The listing builds one solid part. Answer for the finished solid, in the listing's coordinates (mm). Give positions to 0.01 mm unless a question says otherwise; leave off trailing zeros. Loops run counter-clockwise (first coordinate to the right, second up) from the corner with the lowest first, then second, coordinate; pieces in that order, holes last. Notation, with made-up numbers: (6.25, 6) - (61.25, 6) arc R19 cw to (61.25, 14) - close; hole circle Ø10 at (-16.5, 17). An arc over 180 degrees is marked (long way). Write item = value, one per line. Start each with the question number.
1) The part is cut by section A-A on y = 0. Write down the section's boundary in (x, z), plus the area to 3 significant figures.
2) The part is cut by section B-B on x = 0. Write down the section's boundary in (y, z).
3) Consider probe 1 along X at (y, z) = (-0.5, 10.5); probe 2 along Y at (x, z) = (0, -0.8); probe 3 along Z at (x, y) = (69, 3). Determine where each line is inside the solid, lowest interval first.
4) The part is cut by section D-D on x = -21. Write down the section's boundary in (y, z).
5) The part is cut by section C-C on z = 3.5. Write down the section's boundary in (x, y), plus the area to 3 significant figures.
6) Flat-ended cylindrical pins translate along their axes: P1, Ø3, axis at x = 51.5, y = -1, coming from the +Z side; P2, Ø6, axis at x = 32.5, z = 3.5, coming from the -Y side. Find the tip coordinate at first contact, or state that the pin passes through.
from build123d import *

# Parameters (mm, degrees)
BOSS_EXTRUDE1_DEPTH     = 3.5
SKETCH3_R               = 2
CUT_EXTRUDE1_DEPTH      = 7
SKETCH4_R               = 1.5
CUT_EXTRUDE2_DEPTH      = 1
CUT_EXTRUDE2_DEPTH_BACK = 190


with BuildPart() as part:
    # Sketch1 → Boss-Extrude1 (new body, symmetric)
    with BuildSketch(Plane(origin=(0, 0, 0), x_dir=(1, 0, 0), z_dir=(0, 1, 0))):
        Polygon((94.5, 1.75), (94.5, -20), (91, -20), (91, -1.75), (-91, -1.75), (-91, -20), (-94.5, -20), (-94.5, 1.75), align=None)
    extrude(amount=BOSS_EXTRUDE1_DEPTH, both=True)

    # Sketch3 → Cut-Extrude1 (cut)
    with BuildSketch(Plane(origin=(0, 0, -1.75), x_dir=(-1, 0, 0), z_dir=(0, 0, -1))):
        Circle(SKETCH3_R)
    extrude(amount=-CUT_EXTRUDE1_DEPTH, mode=Mode.SUBTRACT)

    # Sketch4 → Cut-Extrude2 (cut, two sides)
    with BuildSketch(Plane.ZY.offset(94.5)) as cut_extrude2_sk:
        with Locations((16.25, 0)):
            Circle(SKETCH4_R)
    extrude(amount=CUT_EXTRUDE2_DEPTH, mode=Mode.SUBTRACT)
    extrude(cut_extrude2_sk.sketch, amount=-CUT_EXTRUDE2_DEPTH_BACK, mode=Mode.SUBTRACT)


solid = part.part
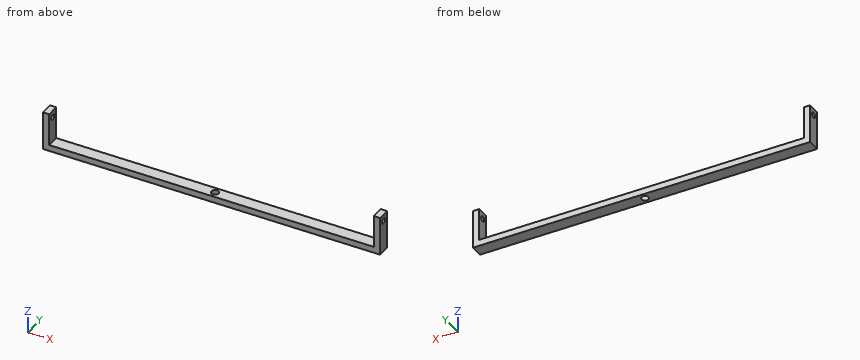
Answer below:
q1.outline = (-94.5, -1.75) - (-2, -1.75) - (-2, 1.75) - (-91, 1.75) - (-91, 14.75) - (-94.5, 14.75) - close; (-94.5, 17.75) - (-91, 17.75) - (-91, 20) - (-94.5, 20) - close; (2, -1.75) - (94.5, -1.75) - (94.5, 14.75) - (91, 14.75) - (91, 1.75) - (2, 1.75) - close; (91, 17.75) - (94.5, 17.75) - (94.5, 20) - (91, 20) - close
q1.area = 754 mm2
q2.outline = (-3.5, -1.75) - (-2, -1.75) - (-2, 1.75) - (-3.5, 1.75) - close; (2, -1.75) - (3.5, -1.75) - (3.5, 1.75) - (2, 1.75) - close
q3.probe_1 = -94.5 to -91, 91 to 94.5
q3.probe_2 = -3.5 to -2, 2 to 3.5
q3.probe_3 = -1.75 to 1.75
q4.outline = (-3.5, -1.75) - (3.5, -1.75) - (3.5, 1.75) - (-3.5, 1.75) - close
q5.outline = (-94.5, -3.5) - (-91, -3.5) - (-91, 3.5) - (-94.5, 3.5) - close; (91, -3.5) - (94.5, -3.5) - (94.5, 3.5) - (91, 3.5) - close
q5.area = 49.0 mm2
q6.P1 = 1.75
q6.P2 = -3.5
